Input: dimensioned drawing with shaded views. Units: mm. Origin: part minimum x, y, z. Round coordinates to 2 decimals unless told otherwise and drop trailing zeros. Write each loop counter-clockwise with the first axis right and the second up, starting at its lowest first coordinate (ties: lowest second). Pieces come first, ordered by that corner, then holes. Notation, with made-up numbers: M 64,-31.75 L 92,-31.75 A14 cw 92,-27.75 Z; hole C 80,-25.5 d3. An arc over 180 degrees is marked long. Answer as CSV lines item,"result". Start each with the question number.
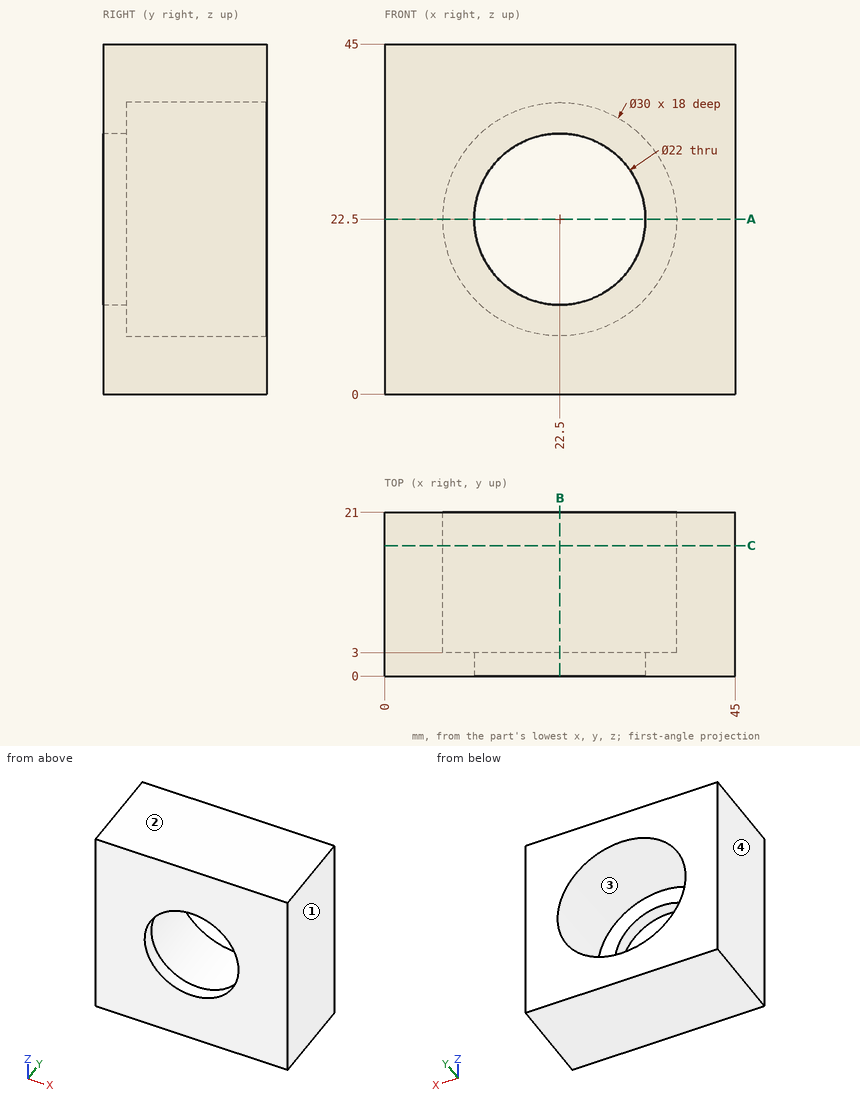
Item 1: Cut plane C-C, the plane y = 16.75. Return loops of the section in (x, z).
Item 2: Cut plane A-A, the plane z = 22.5. Return loops of the section in (x, y), plus the area to 3 significant figures.
Item 3: Cut plane B-B, the plane x = 22.5. Return loops of the section in (y, z).
Item 4: Pin query (flat end, axial travel): pin 1 Ø13 at (x, z) = (22.5, 22.5) entering from +Y. Return the tip coordinate at first contact, or that it passes through.
Item 5: Line query: line 1 (X direction, y = 2.15, z = 22.5); line 2 (X direction, y = 8, z = 22.5); line 3 (Y direction, x = 33.5, z = 13). Output: solid intervals per line, ascending. Write a range as [from, to].
Item 6: Draft query along X for the marked faces 1, 2, 3 and 4. Return one class per face: +X half, -X half, draft (parallel to the pull), parting line (faces both ways), or undercut.
Results list:
1,outline,"M 0,0 L 45,0 L 45,45 L 0,45 Z; hole C 22.5,22.5 d30"
2,outline,"M 0,0 L 11.5,0 L 11.5,3 L 7.5,3 L 7.5,21 L 0,21 Z; M 33.5,0 L 45,0 L 45,21 L 37.5,21 L 37.5,3 L 33.5,3 Z"
2,area,"339 mm²"
3,outline,"M 0,0 L 21,0 L 21,7.5 L 3,7.5 L 3,11.5 L 0,11.5 Z; M 0,33.5 L 3,33.5 L 3,37.5 L 21,37.5 L 21,45 L 0,45 Z"
4,pin 1,"through"
5,line 1,"[0, 11.5], [33.5, 45]"
5,line 2,"[0, 7.5], [37.5, 45]"
5,line 3,"[0, 3]"
6,face 1,"+X half"
6,face 2,"draft"
6,face 3,"undercut"
6,face 4,"-X half"
